Geometry: final body of the model. Coordinates: model frame, mm. A direction names the side the tool comes from. Coordinates: 2 decimals unless noted, no trailing zeros. Order: outer loops, then holes, each group sorted by start corner. A loop starts at its lowest first (then second) coordinate and runs counter-clockwise, first axis right, second up. Notation, with made-up numbers: (45.5, 24.5) -> (96.5, 24.5) arc R19 cw to (96.5, 46.5) -> close; hole circle Ø6 at (88.5, 2.5). An arc over 180 degrees is marked (long way). Answer in a Markdown table with one row per item. Add a question column.
1) Section query A-A on z = -16.5. Return the cut outline in (x, y), then the cut area to 3 significant figures.
2) Section query B-B on y = 1.75. Return the cut outline in (x, z).
3) Contact query for flat-ended pins moving along their axis: P1, Ø5.5, axis at x = 2, y = -0.5, coming from the -Z side; P2, Ø1.5, axis at x = 9.5, y = 0, coming from the +Z side; P3, Ø4.5, axis at y = -6.5, z = 8, coming from the +X side. Output: stop coordinate, or through.
4) Section query D-D on z = 33. Return the cut outline in (x, y), then the cut area to 3 significant figures.
5) Ray query, line 1 (X direction, y = -4.25, z = 3); line 2 (Y direction, x = -2, z = -16); line 3 (Y direction, x = 26, z = -8.5). Return the intervals inside material, ascending. Write a range as from..to.
6) Section query C-C on x = -8. Return the cut outline in (y, z).
7) Set-up query: faces 1 (the face through (12.804, 1.722, -30.172)), 2 (the face through (22.62, 3.63, 31.83)), 3 (the face through (22.62, 3.63, -30.17)), 4 (the face through (12.804, 1.722, 31.828)). Return all of +Z, -Z, +X, -X, +Y, -Y with unobstructed straight access to the full face (end or side cutting, diameter ignored); none if empty.
```python
from build123d import *

# Parameters (mm, degrees)
SKETCH1_W             = 40
SKETCH1_H             = 47
BOSS_EXTRUDE1_DEPTH   = 2
BODY_MOVE_COPY1_ANGLE = 11
SKETCH2_W             = 5
SKETCH2_H             = 10
BOSS_EXTRUDE2_DEPTH   = 46.5
SKETCH4_W             = 10
SKETCH4_H             = 15
BOSS_EXTRUDE3_DEPTH   = 2
SKETCH5_W             = 10
SKETCH5_H             = 15
BOSS_EXTRUDE4_DEPTH   = 2


with BuildPart() as part:
    # Sketch1 → Boss-Extrude1 (new body)
    with BuildSketch(Plane(origin=(0, 0, 0), x_dir=(1, 0, 0), z_dir=(0, 1, 0))):
        with Locations((7.778638156, -0.723210277)):
            Rectangle(SKETCH1_W, SKETCH1_H)
    extrude(amount=BOSS_EXTRUDE1_DEPTH)


with BuildPart() as part_1:
    # Body-Move/Copy1: moved
    add(part.part.rotate(Axis((9.114441417, 1.5, 0), (0, 0, 1)), BODY_MOVE_COPY1_ANGLE))

    # Sketch2 → Boss-Extrude2 (add)
    with BuildSketch(Plane(origin=(0.351616414, 0, 24.223210277), x_dir=(1, 0, 0), z_dir=(0, 0, 1))):
        with Locations((-8.447854102, -7.138980591)):
            Rectangle(SKETCH2_W, SKETCH2_H)
    extrude(amount=-BOSS_EXTRUDE2_DEPTH)

    # Sketch4 → Boss-Extrude3 (add)
    with BuildSketch(Plane(origin=(-0.044520197, 0.229036558, 0), x_dir=(0.9816271834475203, 0.19080899537728402, 0), z_dir=(-0.190808995377284, 0.9816271834475203, 0))):
        with Locations((17.897393689, -31.723210277)):
            Rectangle(SKETCH4_W, SKETCH4_H)
    extrude(amount=-BOSS_EXTRUDE3_DEPTH)

    # Sketch5 → Boss-Extrude4 (add)
    with BuildSketch(Plane(origin=(-0.044520197, 0.229036558, 0), x_dir=(0.9816271834475203, 0.19080899537728402, 0), z_dir=(-0.190808995377284, 0.9816271834475203, 0))):
        with Locations((17.897393689, 30.276789723)):
            Rectangle(SKETCH5_W, SKETCH5_H)
    extrude(amount=-BOSS_EXTRUDE4_DEPTH)


solid = part_1.part
```
Result:
| question | item | result |
|---|---|---|
| 1 | outline | (-11.92, -2.08) -> (-11.54, -4.04) -> (-10.6, -3.86) -> (-10.6, -12.14) -> (-5.6, -12.14) -> (-5.6, -2.89) -> (27.72, 3.59) -> (27.34, 5.55) -> close |
| 1 | area | 124 mm2 |
| 2 | outline | (7.78, -22.78) -> (12.8, -22.78) -> (12.8, -37.78) -> (18.26, -37.78) -> (18.26, 39.22) -> (12.8, 39.22) -> (12.8, 24.22) -> (7.78, 24.22) -> close |
| 3 | P1 | z = -22.78 |
| 3 | P2 | z = 24.22 |
| 3 | P3 | x = -5.6 |
| 4 | outline | (12.62, 2.69) -> (13, 0.73) -> (22.81, 2.63) -> (22.43, 4.6) -> close |
| 4 | area | 20.0 mm2 |
| 5 | line 1 | -10.6..-5.6 |
| 5 | line 2 | -2.19..-0.15 |
| 5 | line 3 | 3.25..5.29 |
| 6 | outline | (-12.14, -22.28) -> (-3.35, -22.28) -> (-3.35, -22.78) -> (-1.32, -22.78) -> (-1.32, 24.22) -> (-12.14, 24.22) -> close |
| 7 | face 1 | -Z, -X, -Y |
| 7 | face 2 | +Z, +X, +Y |
| 7 | face 3 | -Z, +X, +Y |
| 7 | face 4 | +Z, -X, -Y |
